from build123d import *

# Parameters (mm, degrees)
SKETCH1_W           = 29
SKETCH1_H           = 35
BOSS_EXTRUDE1_DEPTH = 17.5
FILLET1_R           = 5
SKETCH2_R           = 17.5
BOSS_EXTRUDE2_DEPTH = 28
SKETCH3_R           = 15
CUT_EXTRUDE1_DEPTH  = 20
CUT_EXTRUDE2_REACH  = 59.771
SKETCH4_R           = 1.5


with BuildPart() as part:
    # Sketch1 → Boss-Extrude1 (new, symmetric)
    with BuildSketch(Plane(origin=(0, 0, 0), x_dir=(1, 0, 0), z_dir=(0, 1, 0))):
        Rectangle(SKETCH1_W, SKETCH1_H)
    extrude(amount=BOSS_EXTRUDE1_DEPTH, both=True)

    # Fillet1
    fillet1_edges = [part.edges().sort_by_distance(p)[0] for p in [
        (-14.5, 0, 17.5),
        (-14.5, 0, -17.5),
    ]]
    fillet(fillet1_edges, radius=FILLET1_R)

    # Sketch2 → Boss-Extrude2 (add)
    with BuildSketch(Plane(origin=(14.5, 0, 0), x_dir=(0, 0, -1), z_dir=(1, 0, 0))):
        Circle(SKETCH2_R)
    extrude(amount=BOSS_EXTRUDE2_DEPTH)

    # Sketch3 → Cut-Extrude1 (cut)
    with BuildSketch(Plane(origin=(42.5, 0, 0), x_dir=(0, 0, -1), z_dir=(1, 0, 0))):
        Circle(SKETCH3_R)
    extrude(amount=-CUT_EXTRUDE1_DEPTH, mode=Mode.SUBTRACT)

    # Sketch4 → Cut-Extrude2 (cut, up to next)
    with BuildSketch(Plane.XZ.offset(17.5), mode=Mode.PRIVATE) as cut_extrude2_sk1:
        with Locations(Location((0, 12.5, 0), (0, 0, 270))):
            Circle(SKETCH4_R)
    cut_extrude2_tool1 = extrude(cut_extrude2_sk1.sketch, amount=-CUT_EXTRUDE2_REACH, mode=Mode.PRIVATE) & part.part
    # Sketch4 → Cut-Extrude2 (cut, up to next)
    with BuildSketch(Plane.XZ.offset(17.5), mode=Mode.PRIVATE) as cut_extrude2_sk2:
        with Locations(Location((10.825317547, 6.25, 0), (0, 0, 270))):
            Circle(SKETCH4_R)
    cut_extrude2_tool2 = extrude(cut_extrude2_sk2.sketch, amount=-CUT_EXTRUDE2_REACH, mode=Mode.PRIVATE) & part.part
    # Sketch4 → Cut-Extrude2 (cut, up to next)
    with BuildSketch(Plane.XZ.offset(17.5), mode=Mode.PRIVATE) as cut_extrude2_sk3:
        with Locations(Location((10.825317547, -6.25, 0), (0, 0, 270))):
            Circle(SKETCH4_R)
    cut_extrude2_tool3 = extrude(cut_extrude2_sk3.sketch, amount=-CUT_EXTRUDE2_REACH, mode=Mode.PRIVATE) & part.part
    # Sketch4 → Cut-Extrude2 (cut, up to next)
    with BuildSketch(Plane.XZ.offset(17.5), mode=Mode.PRIVATE) as cut_extrude2_sk4:
        with Locations(Location((0, -12.5, 0), (0, 0, 270))):
            Circle(SKETCH4_R)
    cut_extrude2_tool4 = extrude(cut_extrude2_sk4.sketch, amount=-CUT_EXTRUDE2_REACH, mode=Mode.PRIVATE) & part.part
    # Sketch4 → Cut-Extrude2 (cut, up to next)
    with BuildSketch(Plane.XZ.offset(17.5), mode=Mode.PRIVATE) as cut_extrude2_sk5:
        with Locations(Location((-10.825317547, -6.25, 0), (0, 0, 270))):
            Circle(SKETCH4_R)
    cut_extrude2_tool5 = extrude(cut_extrude2_sk5.sketch, amount=-CUT_EXTRUDE2_REACH, mode=Mode.PRIVATE) & part.part
    # Sketch4 → Cut-Extrude2 (cut, up to next)
    with BuildSketch(Plane.XZ.offset(17.5), mode=Mode.PRIVATE) as cut_extrude2_sk6:
        with Locations(Location((-10.825317547, 6.25, 0), (0, 0, 270))):
            Circle(SKETCH4_R)
    cut_extrude2_tool6 = extrude(cut_extrude2_sk6.sketch, amount=-CUT_EXTRUDE2_REACH, mode=Mode.PRIVATE) & part.part
    add(cut_extrude2_tool1.solids().sort_by_distance((0, -17.5, 12.5))[0], mode=Mode.SUBTRACT)
    add(cut_extrude2_tool2.solids().sort_by_distance((10.825318, -17.5, 6.25))[0], mode=Mode.SUBTRACT)
    add(cut_extrude2_tool3.solids().sort_by_distance((10.825318, -17.5, -6.25))[0], mode=Mode.SUBTRACT)
    add(cut_extrude2_tool4.solids().sort_by_distance((0, -17.5, -12.5))[0], mode=Mode.SUBTRACT)
    add(cut_extrude2_tool5.solids().sort_by_distance((-10.825318, -17.5, -6.25))[0], mode=Mode.SUBTRACT)
    add(cut_extrude2_tool6.solids().sort_by_distance((-10.825318, -17.5, 6.25))[0], mode=Mode.SUBTRACT)


solid = part.part
Input: part model. Units: mm. Frame: model coordinates. A direction names the side the tool comes from. Round coordinates to 2 decimals unless told otherwise and drop trailing zeros. Loops run counter-clockwise (first coordinate to the right, second up) from the corner with the lowest first, then second, coordinate; pieces in that order, holes last. Notation, with made-up numbers: (60, 83) -> (83, 83) arc R32 ccw to (83, 118) -> close; hole circle Ø10 at (88.25, 41.5). An arc over 180 degrees is marked (long way). Answer as a JSON object with one key per item and string values. Group by question number.
1) Reachability of faces 4 (the flat face through (14.5, 13, 14)), 5 (the cylindrical face through (28.304, -10.648, 13.887)), 6 (the flat face through (14.5, -14, -14)), 7 (the flat face through (14.5, 14, -13)) from +Z, -Z, +X, -X, +Y, -Y: full face, straight path, thin tool, end or side. Return the list, or none.
2) Ray query, L1, parallel to X at y = -2, z = -6.25; L2, parallel to X at y = -16, z = -7; L3, parallel to Y at x = 20.5, z = 10.5. Return the intervals inside material, ascending.
3) Section query B-B on z = 6. Output: boundary loops of the cut face in (x, y).
4) Section query A-A on x = 0. Output: boundary loops of the cut face in (y, z), plus the area to 4 significant figures.
5) Section query C-C on y = 2. Output: boundary loops of the cut face in (x, z).
6) Section query D-D on x = 28. Output: boundary loops of the cut face in (y, z).
7) Pin query (flat end, axial travel): pin 1 (8 mm diameter, centred on x = 32.5, y = -3.5, fed in from +Z); pin 2 (6 mm diameter, centred on y = 3.5, z = 1.5, fed in from +X). Return the tip coordinate at first contact, or that it passes through.
8) Draft query along X for faces 1 (the cylindrical face through (9.91, -0.25, -5.06)), 2 (the flat face through (0, -17.5, 0)), 3 (the flat face through (42.5, 8, -13)). Return one class per face: +X half, -X half, draft (parallel to the pull), parting line (faces both ways), or undercut.
Reply:
{
 "1": {"face 4": "+Z, +X, +Y", "face 5": "+X", "face 6": "-Z, +X, -Y", "face 7": "-Z, +X, +Y"},
 "2": {"L1": "x = -14.5 to -12.33, -9.33 to 9.33, 12.33 to 22.5", "L2": "x = -14.5 to -12.12, -9.53 to 9.53, 12.12 to 42.5", "L3": "y = -14 to 14"},
 "3": {"outline": "(-14.5, -17.5) -> (-12.3, -17.5) -> (-12.3, 17.5) -> (-14.5, 17.5) -> close; (-9.35, -17.5) -> (9.35, -17.5) -> (9.35, 17.5) -> (-9.35, 17.5) -> close; (12.3, -17.5) -> (14.5, -17.5) -> (14.5, -16.44) -> (42.5, -16.44) -> (42.5, -13.75) -> (22.5, -13.75) -> (22.5, 13.75) -> (42.5, 13.75) -> (42.5, 16.44) -> (14.5, 16.44) -> (14.5, 17.5) -> (12.3, 17.5) -> close"},
 "4": {"outline": "(-17.5, -17.5) -> (17.5, -17.5) -> (17.5, -14) -> (-17.5, -14) -> close; (-17.5, -11) -> (17.5, -11) -> (17.5, 11) -> (-17.5, 11) -> close; (-17.5, 14) -> (17.5, 14) -> (17.5, 17.5) -> (-17.5, 17.5) -> close", "area": "1,015 mm2"},
 "5": {"outline": "(-14.5, -12.5) arc R5 ccw to (-9.5, -17.5) -> (14.5, -17.5) -> (14.5, -17.39) -> (42.5, -17.39) -> (42.5, -14.87) -> (22.5, -14.87) -> (22.5, 14.87) -> (42.5, 14.87) -> (42.5, 17.39) -> (14.5, 17.39) -> (14.5, 17.5) -> (-9.5, 17.5) arc R5 ccw to (-14.5, 12.5) -> close; hole circle Ø3 at (-10.83, -6.25); hole circle Ø3 at (-10.83, 6.25); hole circle Ø3 at (0, -12.5); hole circle Ø3 at (0, 12.5); hole circle Ø3 at (10.83, -6.25); hole circle Ø3 at (10.83, 6.25)"},
 "6": {"outline": "circle Ø35 at (0, 0); hole circle Ø30 at (0, 0)"},
 "7": {"pin 1": "stops at z = 17.5", "pin 2": "stops at x = 22.5"},
 "8": {"face 1": "undercut", "face 2": "draft", "face 3": "+X half"}
}
